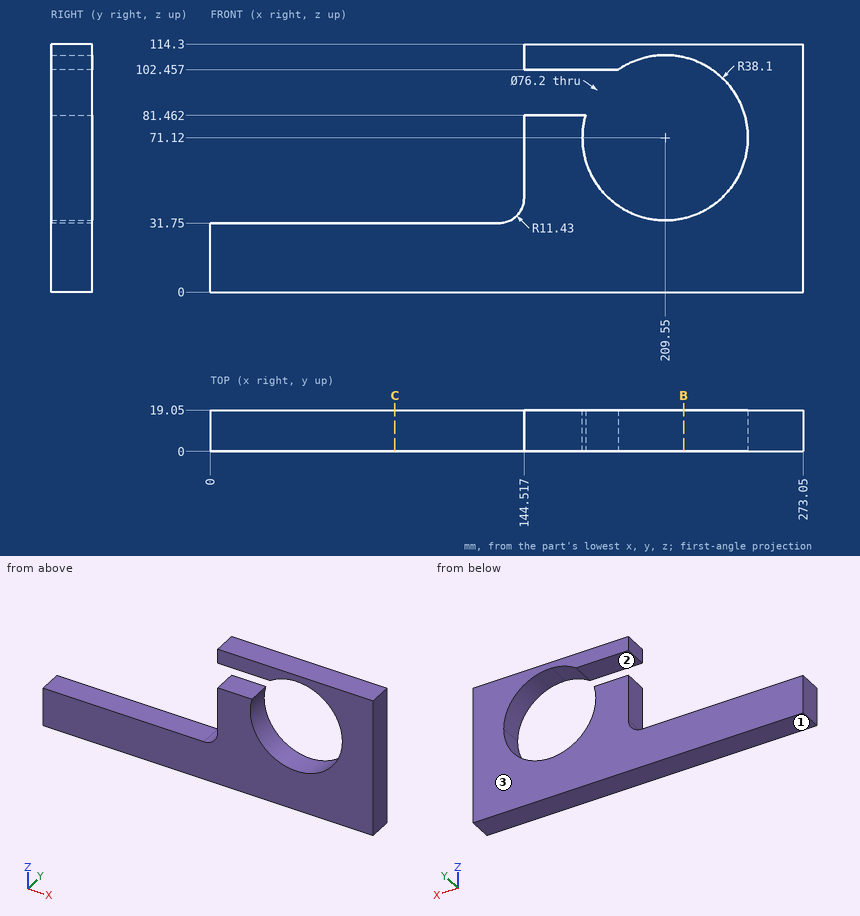
Verification items for this drawing (mm, ordinates from the low corner). Give positions to 0.01 mm unless a question says otherwise; leave off trailing zeros. Order: outer loops, then holes, each group sorted by start corner. A loop starts at its lowest first (then second) coordinate and runs counter-clockwise, first axis right, second up.
1) Cross-section at C-C (x = 85). Record the boundary of the cut face in (y, z), then the cut area to 3 significant figures.
Results are:
outline: (0, 0) - (19.05, 0) - (19.05, 31.75) - (0, 31.75) - close
area: 605 mm2
2) Draft check along Z on the marked faces 1, 2 and 3. Enter one of: released by +Z, released by -Z, zero draft, split by the parting line, or undercut.
Results are:
face 1: released by -Z
face 2: undercut
face 3: zero draft
3) Material ranges on probe 1 along X at (y, z) = (12, 71.12); probe 2 along Z at (x, y) = (209.55, 8); probe 3 along Z at (x, y) = (171, 18), recorded low to high.
Results are:
probe 1: x = 144.52 to 171.45, 247.65 to 273.05
probe 2: z = 0 to 33.02, 109.22 to 114.3
probe 3: z = 0 to 81.46, 102.46 to 114.3
4) Gauge pin test, flat ends, axial feed: pin 1 (9.5 mm diameter, centred on y = 8.5, z = 111.5, fed in from -X); pin 2 (1.5 mm diameter, centred on x = 46.5, y = 15, fed in from +Z). Record the tip position at first contact, or that the pin passes through.
Results are:
pin 1: stops at x = 144.52
pin 2: stops at z = 31.75
5) Cross-section at B-B (x = 218). Record the boundary of the cut face in (y, z), then the cut area to 3 significant figures.
Results are:
outline: (0, 0) - (19.05, 0) - (19.05, 33.97) - (0, 33.97) - close; (0, 108.27) - (19.05, 108.27) - (19.05, 114.3) - (0, 114.3) - close
area: 762 mm2
